from build123d import *

# Parameters (mm, degrees)
F0_R      = 13.85
F1_DEPTH  = 25.3
F2_R      = 1.15
F3_DEPTH  = 12.7
F6_DEPTH  = 25
F7_W      = 1
F7_H      = 2
F8_DEPTH  = 5
F9_R      = 0.75
F10_DEPTH = 24.701


with BuildPart() as f1:
    # F0 (on Top) → F1 (new body)
    with BuildSketch(Plane.XY):
        Circle(F0_R)
    extrude(amount=F1_DEPTH)

    # F2 (on face) → F3 (join)
    with BuildSketch(Plane.XY.offset(25.3)):
        Circle(F2_R)
    extrude(amount=F3_DEPTH)

    # F5 (on offset) → F6 (cut)
    with BuildSketch(Plane.YZ.offset(1.15)):
        Polygon((0, 38.01338), (-1.15913, 38.01338), (-1.216348, 34.017637), (0, 34.017637), align=None)
    extrude(amount=-F6_DEPTH, mode=Mode.SUBTRACT)

    # F7 (on face) → F8 (join)
    with BuildSketch(Plane(origin=(0, 0, 0), x_dir=(1, 0, 0), z_dir=(0, 0, -1))):
        with Locations((-10.35, 1)):
            Rectangle(F7_W, F7_H)
        with Locations((10.35, 1)):
            Rectangle(F7_W, F7_H)
    extrude(amount=F8_DEPTH)

    # F9 (on face) → F10 (cut, through all)
    with BuildSketch(Plane.YZ.offset(10.85)):
        with Locations((-1, -3.5)):
            Circle(F9_R)
    extrude(amount=-F10_DEPTH, mode=Mode.SUBTRACT)


solid = f1.part
For this review, take the finished solid that the model builds, in its own axes (mm). A direction names the side the tool comes from. Round coordinates to 2 decimals unless told otherwise and drop trailing zeros. Write each loop counter-clockwise with the first axis right and the second up, starting at its lowest first coordinate (ties: lowest second). Pieces come first, ordered by that corner, then holes. Notation, with made-up numbers: (30.25, -19.75) - (83.25, -19.75) arc R31 cw to (83.25, 6.25) - close; hole circle Ø1 at (8, 25.25). An arc over 180 degrees is marked (long way). Use a Markdown table: item, result.
Q1. The part is to be moulded in two halves that separate along X. For faces 4 (the cylindrical face through (13.21, 4.16, 12.47)), 5 (the flat face through (10, -1, -5)), 6 (the flat face through (9.85, -1, -2)), say which applies: pulls with the +X half, pulls with the -X half, needs draft (parallel to the pull), parting line crosses it, or undercut.
Derived:
| item | result |
|---|---|
| face 4 | parting line crosses it |
| face 5 | needs draft |
| face 6 | undercut |
Q2. Clearance check with flat-ended pins moving along their axes: pin 1 (1.7 mm diameter, centred on y = -1, z = -3.5, fed in from +X); pin 2 (4 mm diameter, centred on x = -7, z = 14, fed in from +Y); pin 3 (8 mm diameter, centred on x = 0.5, y = 3, fed in from -Z); pin 4 (0.9 mm diameter, centred on y = -1, z = -3.5, fed in from +X). State where each tip first meets the part, or that it passes through.
Derived:
| item | result |
|---|---|
| pin 1 | stops at x = 10.85 |
| pin 2 | stops at y = 12.92 |
| pin 3 | stops at z = 0 |
| pin 4 | passes through |
Q3. Wall thickness on line 1 along Z through (x, y) = (10.45, -1); line 2 along Z through (x, y) = (-4.75, -8); line 3 along X through (y, z) = (-9.5, 16): over which ranges is each line inside the solid? List them lowest first.
Derived:
| item | result |
|---|---|
| line 1 | z = -5 to -4.25, -2.75 to 25.3 |
| line 2 | z = 0 to 25.3 |
| line 3 | x = -10.08 to 10.08 |
Q4. We need section A-A (z = -3.5). Give the boundary of the cut face in (x, y).
Derived:
| item | result |
|---|---|
| outline | (-10.85, -2) - (-9.85, -2) - (-9.85, -1.75) - (-10.85, -1.75) - close; (-10.85, -0.25) - (-9.85, -0.25) - (-9.85, 0) - (-10.85, 0) - close; (9.85, -2) - (10.85, -2) - (10.85, -1.75) - (9.85, -1.75) - close; (9.85, -0.25) - (10.85, -0.25) - (10.85, 0) - (9.85, 0) - close |
Q5. We need section D-D (y = 8.5). Give the boundary of the cut face in (x, z), plus the area to 3 significant figures.
Derived:
| item | result |
|---|---|
| outline | (-10.93, 0) - (10.93, 0) - (10.93, 25.3) - (-10.93, 25.3) - close |
| area | 553 mm2 |
Q6. We need section C-C (z = 30.5). Give the boundary of the cut face in (x, y), plus the area to 3 significant figures.
Derived:
| item | result |
|---|---|
| outline | circle Ø2.3 at (0, 0) |
| area | 4.15 mm2 |
Q7. Machinability: for faces 1 (the flat face through (-10, 0, -2)), 2 (the flat face through (-9.85, -1, -2)), 3 (the flat face through (0, 0, 36)), which of the approach directions +Z, -Z, +X, -X, +Y, -Y give a long, thin tool a straight path to every point of the face, cutting with its end or side? Answer none if there is none.
Derived:
| item | result |
|---|---|
| face 1 | -Z, +X, -X, +Y |
| face 2 | -Z, +Y, -Y |
| face 3 | +Z, +X, -X, -Y |
Q8. We need section B-B (x = 0). Give the boundary of the cut face in (y, z), plus the area to 3 significant figures.
Derived:
| item | result |
|---|---|
| outline | (-13.85, 0) - (13.85, 0) - (13.85, 25.3) - (1.15, 25.3) - (1.15, 38) - (0, 38) - (0, 34.02) - (-1.15, 34.02) - (-1.15, 25.3) - (-13.85, 25.3) - close |
| area | 725 mm2 |
